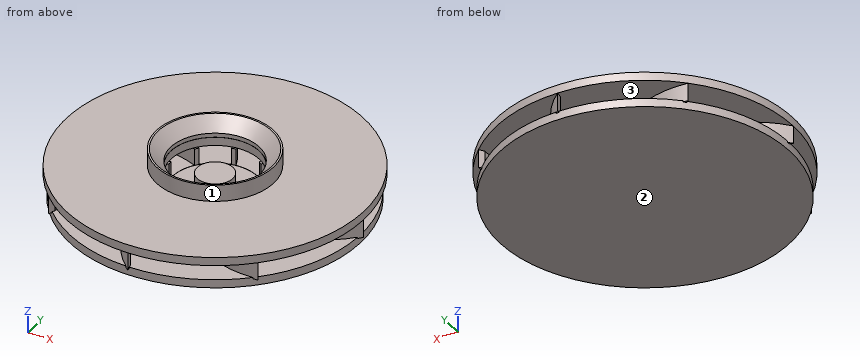
from build123d import *

# Parameters (mm, degrees)
F0_R      = 35
F1_DEPTH  = 2
F2_R      = 5
F3_DEPTH  = 4
F4_W      = 1.5
F4_H      = 8.0229806336
F7_COUNT  = 8
F8_W      = 26.6654435545
F8_H      = 7.6421163976
F10_R     = 35.7945573746
F10_R_2   = 10.639493897
F11_DEPTH = 2
F12_R     = 7.8850304464
F13_DEPTH = 25
F14_R     = 14.11317868
F14_R_2   = 10.6813839673
F15_DEPTH = 4
F16_SIZE  = 3


with BuildPart() as f1:
    # F0 (on Top) → F1 (new body)
    with BuildSketch(Plane.XY):
        Circle(F0_R)
    extrude(amount=F1_DEPTH)



with BuildPart() as f3:
    # F2 (on face) → F3 (new body)
    with BuildSketch(Plane.XY.offset(2)):
        Circle(F2_R)
    extrude(amount=F3_DEPTH)


with BuildPart() as f6:
    # F6: sweep along a path in F5
    with BuildLine(Plane.XY) as f6_path:
        ThreePointArc((0, 0), (-8.1347441665, -17.5274070352), (0, -35.0548140705))
    # F4 (on Front) → F6 (sweep)
    with BuildSketch(Plane.XZ):
        with Locations((0, 5.7041863911)):
            Rectangle(F4_W, F4_H)
    sweep(path=f6_path.line)


with BuildPart() as f1_1:
    add(f1.part)

    add(f3.part)  # F7 merges F3

    add(f6.part)  # F7 merges F6
    # F7: F6 ×8 about axis
    f7_axis = Axis((0, 0, 6), (0, 0, 1))
    for i in range(1, F7_COUNT):
        add(f6.part.rotate(f7_axis, i * 360 / F7_COUNT))

    # F8 (on Front) → F9 (revolve, cut)
    with BuildSketch(Plane.XZ):
        with Locations((23.4964704141, 9.8134223372)):
            Rectangle(F8_W, F8_H)
        Polygon((10.1637486368, 5.9923641384), (10.1637486368, 13.634480536), (4.3031405658, 13.634480536), (4.3031405658, 1.9518490881), (10.1637486368, 1.9518490881), align=None)
    revolve(axis=Axis((0, 0, 0), (0, 0, 1)), mode=Mode.SUBTRACT)

    # F10 (on face) → F11 (join)
    with BuildSketch(Plane.XY.offset(5.9923641384)):
        Circle(F10_R)
        Circle(F10_R_2, mode=Mode.SUBTRACT)
    extrude(amount=F11_DEPTH)

    # F12 (on face) → F13 (cut)
    with BuildSketch(Plane.XY.offset(6)):
        Circle(F12_R)
        with BuildLine():
            ThreePointArc((-0.4521737471, -4.2793174258), (-1.6150666235, -3.9885559455), (-2.6526354387, -3.3882951404))
            ThreePointArc((-2.6526354387, -3.3882951404), (-1.6440902169, -2.2260491927), (-0.5583723561, -1.1355466324))
            ThreePointArc((-0.5583723561, -1.1355466324), (-0.5580653725, -2.7092153878), (-0.4521737471, -4.2793174258))
        make_face(mode=Mode.SUBTRACT)
        with BuildLine():
            ThreePointArc((-3.3456694935, -2.7061992478), (-3.9623595177, -1.6783103947), (-4.2715829771, -0.5201899637))
            ThreePointArc((-4.2715829771, -0.5201899637), (-2.7366018207, -0.4115071382), (-1.1977816036, -0.4081238447))
            ThreePointArc((-1.1977816036, -0.4081238447), (-2.3103163817, -1.5210927632), (-3.3456694935, -2.7061992478))
        make_face(mode=Mode.SUBTRACT)
        with BuildLine():
            ThreePointArc((2.7061992478, -3.3456694935), (1.6783103947, -3.9623595177), (0.5201899637, -4.2715829771))
            ThreePointArc((0.5201899637, -4.2715829771), (0.4115071382, -2.7366018207), (0.4081238447, -1.1977816036))
            ThreePointArc((0.4081238447, -1.1977816036), (1.5210927632, -2.3103163817), (2.7061992478, -3.3456694935))
        make_face(mode=Mode.SUBTRACT)
        with BuildLine():
            ThreePointArc((4.2793174258, -0.4521737471), (3.9885559455, -1.6150666235), (3.3882951404, -2.6526354387))
            ThreePointArc((3.3882951404, -2.6526354387), (2.2260491927, -1.6440902169), (1.1355466324, -0.5583723561))
            ThreePointArc((1.1355466324, -0.5583723561), (2.7092153878, -0.5580653725), (4.2793174258, -0.4521737471))
        make_face(mode=Mode.SUBTRACT)
        with BuildLine():
            ThreePointArc((-4.2793174258, 0.4521737471), (-3.9885559455, 1.6150666235), (-3.3882951404, 2.6526354387))
            ThreePointArc((-3.3882951404, 2.6526354387), (-2.2260491927, 1.6440902169), (-1.1355466324, 0.5583723561))
            ThreePointArc((-1.1355466324, 0.5583723561), (-2.7092153878, 0.5580653725), (-4.2793174258, 0.4521737471))
        make_face(mode=Mode.SUBTRACT)
        with BuildLine():
            ThreePointArc((-2.7061992478, 3.3456694935), (-1.6783103947, 3.9623595177), (-0.5201899637, 4.2715829771))
            ThreePointArc((-0.5201899637, 4.2715829771), (-0.4115071382, 2.7366018207), (-0.4081238447, 1.1977816036))
            ThreePointArc((-0.4081238447, 1.1977816036), (-1.5210927632, 2.3103163817), (-2.7061992478, 3.3456694935))
        make_face(mode=Mode.SUBTRACT)
        with BuildLine():
            ThreePointArc((3.3456694935, 2.7061992478), (3.9623595177, 1.6783103947), (4.2715829771, 0.5201899637))
            ThreePointArc((4.2715829771, 0.5201899637), (2.7366018207, 0.4115071382), (1.1977816036, 0.4081238447))
            ThreePointArc((1.1977816036, 0.4081238447), (2.3103163817, 1.5210927632), (3.3456694935, 2.7061992478))
        make_face(mode=Mode.SUBTRACT)
        with BuildLine():
            ThreePointArc((0.4521737471, 4.2793174258), (1.6150666235, 3.9885559455), (2.6526354387, 3.3882951404))
            ThreePointArc((2.6526354387, 3.3882951404), (1.6440902169, 2.2260491927), (0.5583723561, 1.1355466324))
            ThreePointArc((0.5583723561, 1.1355466324), (0.5580653725, 2.7092153878), (0.4521737471, 4.2793174258))
        make_face(mode=Mode.SUBTRACT)
    extrude(amount=F13_DEPTH, mode=Mode.SUBTRACT)

    # F14 (on face) → F15 (join)
    with BuildSketch(Plane.XY.offset(7.9923641384)):
        Circle(F14_R)
        Circle(F14_R_2, mode=Mode.SUBTRACT)
    extrude(amount=F15_DEPTH)

    # F16
    f16_edges = [f1_1.edges().sort_by_distance(p)[0] for p in [
        (-10.681384, 0, 11.992364),
    ]]
    chamfer(f16_edges, length=F16_SIZE)


solid = f1_1.part
Here's how the part is built. I have some questions about the finished solid (model axes, mm). Face numbers are marked on the shaded views. Round coordinates to 2 decimals unless told otherwise and drop trailing zeros. Order: outer loops, then holes, each group sorted by start corner. A loop starts at its lowest first (then second) coordinate and runs counter-clockwise, first axis right, second up. Notation, with made-up numbers: M 23,75 L 36,75 A28 ccw 36,98 Z; hole C 27,82.5 d10. An arc over 180 degrees is marked long. Return JSON: item names as keys, results as strings. Group by question number.
1. If we section it at A-A on z = 3.5: State how many separate pieces and enclosed holes the cut face has, then the cut area to 3 significant figures.
2. If we section it at B-B on y = -18: List the corners of the cut face in (x, z) for me.
3. Please list where these lines run through material, in increasing order: probe 1 along Z at (x, y) = (10, 32.5); probe 2 along X at (y, z) = (-17, 5); probe 3 along Y at (x, z) = (0, 7.15).
4. I'm going to push flat-ended pins straight in: pin 1 Ø12 at (x, y) = (19.5, -16.5) entering from +Z; pin 2 Ø0.7 at (x, y) = (1.5, -10.5) entering from +Z; pin 3 Ø5 at (x, z) = (-0.5, 3) entering from -Y; pin 4 Ø17 at (x, y) = (0, 0) entering from +Z. Where does each tip first touch, or does it pass through?
5. If we section it at D-D on y = -30: List the corners of the cut face in (x, z) for me.
6. If we mould it in two halves opening along Y, with no side actions, what happens to the marked faces 1, 2 and 3? For each: pulls with the +Y half, pulls with the -Y half, needs draft (parallel to the pull), parting line crosses it, or undercut.
7. If we section it at C-C on x = -30.5: List the corners of the cut face in (y, z) for me (3 decimals).
Reply:
{
 "1": {"separate pieces": "9", "enclosed holes": "0", "area": "288 mm^2"},
 "2": {"outline": "M -30.94,5.99 L -24.85,5.99 L -24.85,2 L -30.02,2 L -30.02,0 L 30.02,0 L 30.02,2 L 7.17,2 L 7.17,5.99 L 30.94,5.99 L 30.94,7.99 L -30.94,7.99 Z; hole M -23.86,2 L -8.62,2 L -8.62,5.99 L -23.86,5.99 Z; hole M -7.65,2 L 5.82,2 L 5.82,5.99 L -7.65,5.99 Z"},
 "3": {"probe 1": "0 to 2, 5.99 to 7.99", "probe 2": "-24.61 to -23.61, -8.62 to -7.65, 4.92 to 6.21", "probe 3": "-35.79 to -10.64, 10.64 to 35.79"},
 "4": {"pin 1": "z = 7.99", "pin 2": "z = 9.27", "pin 3": "y = -35.79", "pin 4": "z = 6"},
 "5": {"outline": "M -19.53,5.99 L -5.03,5.99 L -5.03,2 L -18.03,2 L -18.03,0 L 18.03,0 L 18.03,2 L -3.88,2 L -3.88,5.99 L 19.53,5.99 L 19.53,7.99 L -19.53,7.99 Z"},
 "6": {"face 1": "parting line crosses it", "face 2": "needs draft", "face 3": "undercut"},
 "7": {"outline": "M -18.735,5.992 L 3.536,5.992 L 3.536,2 L -17.168,2 L -17.168,0 L 17.168,0 L 17.168,2 L 4.709,2 L 4.709,5.992 L 18.735,5.992 L 18.735,7.992 L -18.735,7.992 Z"}
}
